Read the model definition and answer for the solid it produces. Units are mm, in the model's axes. A direction names the side the tool comes from. Round coordinates to 2 decimals unless told otherwise and drop trailing zeros. Write each loop counter-clockwise with the first axis right and the second up, starting at its lowest first coordinate (ties: lowest second). Pieces come first, ordered by that corner, then holes. Notation, with made-up numbers: (-0.75, -10) - (30.25, -10) arc R23 ccw to (30.25, 26) - close; hole circle Ø3 at (15.5, -31). An arc over 180 degrees is marked (long way). One line per item, written item: value. Start each with the question number.
(1) Find the intervals of material crossed by L1, parallel to Y at x = -469, z = -42; L2, parallel to Z at x = -443, y = 58.5, in increasing order.
(2) A flat-ended cylindrical pin translates along its axis: pin 1 Ø5 at (x, y) = (-462, -34) entering from -Z. Find the tip coordinate at first contact, or state that the pin passes through.
(3) A cutting plane is placed at B-B, the plane x = -416. Determine the outline of the cut face in (y, z), plus the area to 3 significant figures.
(4) The mould has two halves that part along Y. Classify faces 1 (the face through (-443, 11, 0)), 2 (the face through (-441, -139.329, -103)), 3 (the face through (-443, 158.671, -100)): +Y half, -Y half, draft (parallel to the pull), parting line (faces both ways), or undercut.
(5) A cutting plane is placed at C-C, the plane y = 15. Determine the outline of the cut face in (x, z), plus the area to 3 significant figures.
(6) For faces 4 (the face through (-443, 11, -2)), 5 (the face through (-441, -141.329, -100)), determine the directions among +Z, -Z, +X, -X, +Y, -Y from which every point of the face is accessible in a straight line to the end or side of a thin tool.
(7) A cutting plane is placed at A-A, the plane z = -38. Determine the outline of the cut face in (x, y).
from build123d import *

# Parameters (mm, degrees)
SKETCH1_W                    = 140
SKETCH1_H                    = 300
BASE_FLANGE1_DEPTH           = 2
EDGE_FLANGE1_STRIP_W         = 9.4732
EDGE_FLANGE1_STRIP_H         = 2
EDGE_FLANGE1_STRIP_CUT_DEPTH = 140
EDGE_FLANGE1_DEPTH           = 140
EDGE_FLANGE2_STRIP_W         = 9.4732
EDGE_FLANGE2_STRIP_H         = 2
EDGE_FLANGE2_STRIP_CUT_DEPTH = 140
EDGE_FLANGE2_DEPTH           = 140


# Sheet-metal steps are written as plain solids
with BuildPart() as part:
    # Sketch1 → Base-Flange1 (new body)
    with BuildSketch(Plane.XY):
        with Locations((-441.560693642, 8.670520231)):
            Rectangle(SKETCH1_W, SKETCH1_H)
    extrude(amount=-BASE_FLANGE1_DEPTH)

    # Edge-Flange1 strip (across the edge) → Edge-Flange1 strip cut (cut)
    with BuildSketch(Plane(origin=(-511.560693642, 158.670520231, -2), x_dir=(0, -1, 0), z_dir=(1, 0, 0))):
        with Locations((-2, -1)):
            Rectangle(EDGE_FLANGE1_STRIP_W, EDGE_FLANGE1_STRIP_H)
    extrude(amount=EDGE_FLANGE1_STRIP_CUT_DEPTH, mode=Mode.SUBTRACT)

    # Edge-Flange1 section (across the edge) → Edge-Flange1 (add)
    with BuildSketch(Plane(origin=(-511.560693642, 158.670520231, -2), x_dir=(0, -1, 0), z_dir=(1, 0, 0))):
        with BuildLine():
            Line((0, 0.7366), (0, 198))
            Line((0, 198), (2, 198))
            Line((2, 198), (2, 0.7366))
            ThreePointArc((2, 0.7366), (2.215745145, 0.215745145), (2.7366, 0))
            Line((2.7366, 0), (2.7366, -2))
            ThreePointArc((2.7366, -2), (0.801531583, -1.198468417), (0, 0.7366))
        make_face()
    extrude(amount=EDGE_FLANGE1_DEPTH)

    # Edge-Flange2 strip (across the edge) → Edge-Flange2 strip cut (cut)
    with BuildSketch(Plane(origin=(-371.560693642, -141.329479769, -2), x_dir=(0, 1, 0), z_dir=(-1, 0, 0))):
        with Locations((-2, -1)):
            Rectangle(EDGE_FLANGE2_STRIP_W, EDGE_FLANGE2_STRIP_H)
    extrude(amount=EDGE_FLANGE2_STRIP_CUT_DEPTH, mode=Mode.SUBTRACT)

    # Edge-Flange2 section (across the edge) → Edge-Flange2 (add)
    with BuildSketch(Plane(origin=(-371.560693642, -141.329479769, -2), x_dir=(0, 1, 0), z_dir=(-1, 0, 0))):
        with BuildLine():
            Line((0, 0.7366), (0, 198))
            Line((0, 198), (2, 198))
            Line((2, 198), (2, 0.7366))
            ThreePointArc((2, 0.7366), (2.215745145, 0.215745145), (2.7366, 0))
            Line((2.7366, 0), (2.7366, -2))
            ThreePointArc((2.7366, -2), (0.801531583, -1.198468417), (0, 0.7366))
        make_face()
    extrude(amount=EDGE_FLANGE2_DEPTH)


solid = part.part
Here are the results:
1. L1: -141.33 to -139.33, 156.67 to 158.67
1. L2: -2 to 0
2. pin 1: z = -2
3. outline: (-141.33, -200) - (-139.33, -200) - (-139.33, -2.74) arc R0.74 cw to (-138.59, -2) - (155.93, -2) arc R0.74 cw to (156.67, -2.74) - (156.67, -200) - (158.67, -200) - (158.67, -2.74) arc R2.74 ccw to (155.93, 0) - (-138.59, 0) arc R2.74 ccw to (-141.33, -2.74) - close
3. area: 1,390 mm²
4. face 1: draft
4. face 2: undercut
4. face 3: +Y half
5. outline: (-511.56, -2) - (-371.56, -2) - (-371.56, 0) - (-511.56, 0) - close
5. area: 280 mm²
6. face 4: -Z, +X, -X
6. face 5: +Z, -Z, +X, -X, -Y
7. outline: (-511.56, -141.33) - (-371.56, -141.33) - (-371.56, -139.33) - (-511.56, -139.33) - close; (-511.56, 156.67) - (-371.56, 156.67) - (-371.56, 158.67) - (-511.56, 158.67) - close
